from build123d import *

# Parameters (mm, degrees)
F0_R     = 5
F1_DEPTH = 3
F2_R     = 10
F3_R     = 5


with BuildPart() as f1:
    # F0 (on Front) → F1 (new body)
    with BuildSketch(Plane.XZ):
        with BuildLine():
            ThreePointArc((-18.427902, 138.781888), (-0.24164, 139.999791), (17.948718, 138.844674))
            Line((17.948718, 138.844674), (18, 159.789056))
            Line((18, 159.789056), (0, 159.789056))
            Line((0, 159.789056), (-5, 159.789056))
            Line((-5, 159.789056), (-19.489739, 146.778655))
            Line((-19.489739, 146.778655), (-18.427902, 138.781888))
        make_face()
        with Locations((0, 147)):
            Circle(F0_R, mode=Mode.SUBTRACT)
    extrude(amount=F1_DEPTH)

    # F2
    f2_edges = [f1.edges().sort_by_distance(p)[0] for p in [
        (18, -1.5, 159.789056),
        (-5, -1.5, 159.789056),
    ]]
    fillet(f2_edges, radius=F2_R)

    # F3
    f3_edges = [f1.edges().sort_by_distance(p)[0] for p in [
        (-19.489739, -1.5, 146.778655),
    ]]
    fillet(f3_edges, radius=F3_R)


solid = f1.part
Design review of the part built by this model. Coordinates are the model's own, in mm. Coordinates: 2 decimals unless noted, no trailing zeros. Loops run counter-clockwise (first coordinate to the right, second up) from the corner with the lowest first, then second, coordinate; pieces in that order, holes last.
Item 1: Add section B-B (y = -2.5). Write out the cut boundary in (x, z).
Completed:
outline: (-19.14, 144.16) - (-18.43, 138.78) arc R140 cw to (17.95, 138.84) - (17.98, 149.76) arc R10 ccw to (7.98, 159.79) - (-1.17, 159.79) arc R10 ccw to (-7.85, 157.23) - (-17.53, 148.54) arc R5 ccw to start; hole circle Ø10 at (0, 147)
Item 2: Add section A-A (x = 0). Write out the cut boundary in (y, z).
Completed:
outline: (-3, 140) - (0, 140) - (0, 142) - (-3, 142) - close; (-3, 152) - (0, 152) - (0, 159.79) - (-3, 159.79) - close
Item 3: Wall thickness on L1, parallel to Z at x = 0, y = -1.4; L2, parallel to X at y = -2.3, z = 151.5; L3, parallel to X at y = -0.5, z = 146.25: over which ranges is each line inside the solid? List them lowest first.
Completed:
L1: z = 140 to 142, 152 to 159.79
L2: x = -14.23 to -2.18, 2.18 to 17.83
L3: x = -18.98 to -4.94, 4.94 to 17.97
Item 4: Add section C-C (z = 151). Write out the cut boundary in (x, y).
Completed:
outline: (-14.79, -3) - (-3, -3) - (-3, 0) - (-14.79, 0) - close; (3, -3) - (17.9, -3) - (17.9, 0) - (3, 0) - close
Item 5: Clearance check with flat-ended pins moving along their axes: pin 1 (3 mm diameter, centred on x = -11.5, z = 154, fed in from +Y); pin 2 (8 mm diameter, centred on x = 0, z = 147, fed in from -Y). State where each tip first meets the part, or that it passes through.
Completed:
pin 1: stops at y = 0
pin 2: passes through
Item 6: Draft analysis for pull direction X (two halves, no side actions). For faces 1 (the flat face through (-12.621, -1.479, 152.946)), 2 (the cylindrical face through (0, -1, 140)), 3 (the cylindrical face through (15.133, -1.521, 156.773)), state which applies: pulls with the +X half, pulls with the -X half, needs draft (parallel to the pull), parting line crosses it, or undercut.
Completed:
face 1: pulls with the -X half
face 2: undercut
face 3: pulls with the +X half
Item 7: Add section D-D (z = 156). Write out the cut boundary in (x, y).
Completed:
outline: (-9.22, -3) - (15.81, -3) - (15.81, 0) - (-9.22, 0) - close
